Autodesk Inventor part; units mm, degrees
ref_plane "YZ Plane" through (0, 0, 0) normal (1, 0, 0) x (0, 1, 0)
ref_plane "XZ Plane" through (0, 0, 0) normal (0, 1, 0) x (-1, 0, 0)
ref_plane "XY Plane" through (0, 0, 0) normal (0, 0, 1) x (1, 0, 0)
sketch "Sketch1" plane through (0, 0, 0) normal (0, 1, 0) x (-1, 0, 0)
  line L0 (0, 0) -> (50.5, 0)
  line L1 (50.5, 0) -> (50.5, -80)
  line L2 (50.5, -80) -> (0, -80)
  line L3 (0, -80) -> (0, 0)
  line L4 (0, -80) -> (9.1, -80)
  line L5 (0, -80) -> (10, -80)
  line L6 (10, -80) -> (10, -50)
  circle A0 centre (10, -30) radius 2.5
  circle A1 centre (10, -50) radius 2.5
  line L7 (9.1, -65.7) -> (9.1, -63.6)
  circle A2 centre (9.1, -16.4) radius 2.1
  circle A3 centre (9.1, -63.6) radius 2.1
  line L8 (0, 0) -> (0, -40)
  line L9 (9.1, -40) -> (32.5, -40)
  circle A4 centre (32.5, -40) radius 5.6
  line L10 (0, 0) -> (0, -10)
  line L11 (30, -10) -> (30, -70)
  circle A5 centre (30, -10) radius 2.5
  circle A6 centre (30, -70) radius 2.5
  line L12 (27.5, -10) -> (30, -10)
  line L13 (9.1, 0) -> (9.1, -10)
  line L14 (9.1, -14.3) -> (9.1, -16.4)
  line L15 (9.1, -10) -> (9.1, 0)
  line L16 (9.1, -18.5) -> (9.1, -14.3)
  line L17 (10, -18.2974) -> (10, -14.5026)
  line L18 (10, -50) -> (10, -47.5)
  line L19 (10, -32.5) -> (10, -30)
  line L20 (9.1, -32.3324) -> (9.1, -27.6676)
  line L21 (10, -80) -> (10, -47.5)
  line L22 (10, -40) -> (10, -27.5)
  line L23 (9.1, -65.7) -> (9.1, -61.5)
  line L24 (9.1, -52.3324) -> (9.1, -47.6676)
  dimension "d17" = 5
  dimension "d0" = 50.5
  dimension "d1" = 80
  dimension "d2" = 9.1
  dimension "d3" = 10
  dimension "d4" = 30
  dimension "d5" = 20
  dimension "d6" = 5
  dimension "d7" = 5
  dimension "d8" = 16.4
  dimension "d9" = 16.4
  dimension "d10" = 4.2
  dimension "d11" = 4.2
  dimension "d12" = 32.5
  dimension "d13" = 11.2
  dimension "d14" = 10
  dimension "d15" = 30
  dimension "d16" = 60
  dimension "d27" = 47.2
extrude "Extrusion1" add sketch "Sketch1" along normal blind 12
sketch "Sketch2" plane through (-50.5, 0, -80) normal (-1, 0, 0) x (0, 0, 1)
  line L0 (80, 0) -> (80, 12)
  line L1 (80, 0) -> (40, 0)
  line L2 (0, 0) -> (80, 0)
  line L3 (40, 0) -> (49.9, 0)
  line L4 (49.9, 0) -> (30.1, 0)
  line L5 (30.1, 0) -> (30.1, 6)
  line L6 (30.1, 6) -> (49.9, 6)
  circle A0 centre (49.9, 6) radius 2.1
  circle A1 centre (30.1, 6) radius 2.1
  dimension "d20" = 9.9
  dimension "d21" = 19.8
  dimension "d22" = 6
  dimension "d23" = 4.2
  dimension "d24" = 4.2
extrude "Extrusion2" cut sketch "Sketch2" against normal blind 7
sketch "Sketch3" plane through (-50.5, 0, -80) normal (-1, 0, 0) x (0, 0, 1)
  circle A0 centre (30.1, 6) radius 2.1
  circle A1 centre (49.9, 6) radius 2.1
  line L0 (0, 0) -> (80, 0)
  line L1 (80, 0) -> (80, 12)
  line L2 (0, 12) -> (80, 12)
  line L3 (0, 0) -> (0, 12)
properties part number "tapaperfil"
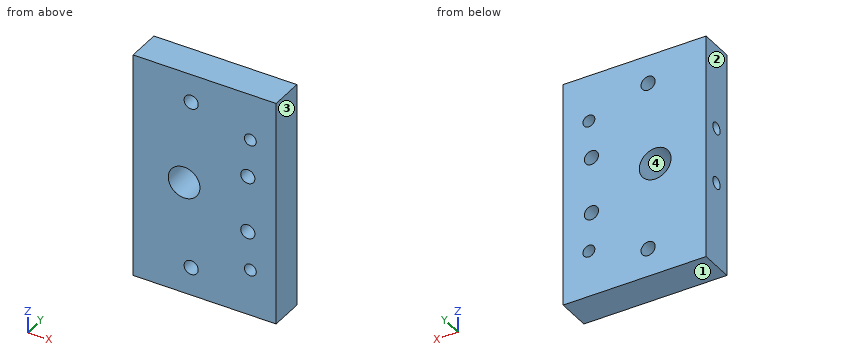
Part model, mm, in its own coordinate system. Face numbers are marked on the shaded views. Coordinates: 2 decimals unless noted, no trailing zeros. Loops run counter-clockwise (first coordinate to the right, second up) from the corner with the lowest first, then second, coordinate; pieces in that order, holes last. Notation, with made-up numbers: M 45.5,-7.5 L 98.5,-7.5 A20 ccw 98.5,19.5 Z; hole C 22.25,11 d8. An arc over 180 degrees is marked long. Use a Markdown table: item, result. Add a question column.
Q1. Cut at B-B (y = 10). Write the cut outline in (x, z).
Q2. Pin check, flat tips, straight feed: P1, Ø3.5, axis at x = -9.1, z = -16.4, coming from the +Y side; P2, Ø2, axis at y = 6, z = -30.5, coming from the -X side. Stop position of each tip, or through.
Q3. Cut at D-D (y = 4.75). Write the cut outline in (x, z), and give its area (3 significant figures).
Q4. Cut at C-C (z = -10). Write the cut outline in (x, y), and give its area (3 significant figures).
Q5. Mould opens along X. For the marked faces 1, 2, 3 and 4 say: +X half, -X half, draft (parallel to the pull), parting line (faces both ways), or undercut.
Q6. Cut at A-A (z = -40). Write the cut outline in (x, y), and give its area (3 significant figures).
Q7. Probe L1, parallel to Z at x = -45, y = 6; L2, parallel to Z at x = -30, y = 7.75; L3, parallel to X at y = 7.5, z = -50. List the from-to ranges inside material, lowest first.
Worked out:
| question | item | result |
|---|---|---|
| 1 | outline | M -50.5,-80 L 0,-80 L 0,0 L -50.5,0 Z; hole C -32.5,-40 d11.2; hole C -30,-70 d5; hole C -30,-10 d5; hole C -10,-50 d5; hole C -10,-30 d5; hole C -9.1,-63.6 d4.2; hole C -9.1,-16.4 d4.2 |
| 2 | P1 | passes through |
| 2 | P2 | stops at x = -43.5 |
| 3 | outline | M -50.5,-80 L 0,-80 L 0,0 L -50.5,0 L -50.5,-28.41 L -43.5,-28.41 L -43.5,-31.79 L -50.5,-31.79 L -50.5,-48.21 L -43.5,-48.21 L -43.5,-51.59 L -50.5,-51.59 Z; hole C -32.5,-40 d11.2; hole C -30,-70 d5; hole C -30,-10 d5; hole C -10,-50 d5; hole C -10,-30 d5; hole C -9.1,-63.6 d4.2; hole C -9.1,-16.4 d4.2 |
| 3 | area | 3,790 mm2 |
| 4 | outline | M -50.5,0 L -32.5,0 L -32.5,12 L -50.5,12 Z; M -27.5,0 L 0,0 L 0,12 L -27.5,12 Z |
| 4 | area | 546 mm2 |
| 5 | face 1 | draft |
| 5 | face 2 | -X half |
| 5 | face 3 | +X half |
| 5 | face 4 | undercut |
| 6 | outline | M -50.5,0 L -38.1,0 L -38.1,12 L -50.5,12 Z; M -26.9,0 L 0,0 L 0,12 L -26.9,12 Z |
| 6 | area | 472 mm2 |
| 7 | L1 | z = -80 to -52, -47.8 to -32.2, -28 to 0 |
| 7 | L2 | z = -80 to -72.5, -67.5 to -45.01, -34.99 to -12.5, -7.5 to 0 |
| 7 | L3 | x = -43.5 to -12.5, -7.5 to 0 |
